Geometry check sheet. Reference: the model listing, model coordinates, mm. Face numbers are marked on the shaded views. A direction names the side the tool comes from. Round coordinates to 2 decimals unless told otherwise and drop trailing zeros. Loops run counter-clockwise (first coordinate to the right, second up) from the corner with the lowest first, then second, coordinate; pieces in that order, holes last. Notation, with made-up numbers: M 77,-33.5 L 133,-33.5 A24 cw 133,-21.5 Z; hole C -24,23 d5. An arc over 180 degrees is marked long. Use one line per item in the form item = value. Start each with the question number.
1. Cross-section at C-C (z = -2.5). Record the boundary of the cut face in (x, y).
2. Cross-section at B-B (y = 3.5). Record the boundary of the cut face in (x, z).
3. Set-up check for the marked faces 1 and 2: record each of +Z, -Z, +X, -X, +Y, -Y from which the full face is reachable in a straight line by a thin tool's end or side.
4. Go/stop test with flat-tipped pins: pin 1 (1.5 mm diameter, centred on x = 26, y = 11.5, fed in from -Z); pin 2 (6 mm diameter, centred on x = 131.5, z = -43.5, fed in from -Y); pin 3 (4 mm diameter, centred on x = 185.5, y = 12.7, fed in from +Z); pin 4 (2 mm diameter, centred on x = 58.5, y = -24, fed in from -Z). Record where each tip stops, or that it passes through.
5. Material ranges on line 1 (X direction, y = 12, z = 3); line 2 (X direction, y = -23, z = -42); line 3 (Y direction, x = 44.5, z = -7), recorded low to high.
6. Cross-section at A-A (x = 93). Record the boundary of the cut face in (y, z), then the cut area to 3 significant figures.
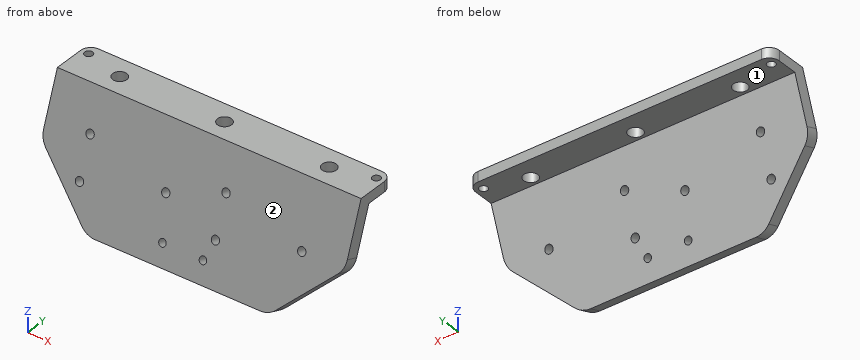
Autodesk Inventor part; units mm, degrees
ref_plane "YZ Plane" through (0, 0, 0) normal (1, 0, 0) x (0, 1, 0)
ref_plane "XZ Plane" through (0, 0, 0) normal (0, 1, 0) x (-1, 0, 0)
ref_plane "XY Plane" through (0, 0, 0) normal (0, 0, 1) x (1, 0, 0)
sketch "Sketch1" plane through (0, 0, 0) normal (0, 0, 1) x (1, 0, 0)
  line L0 (0, 0) -> (190.5, 0)
  line L1 (190.5, 0) -> (190.5, 19.05)
  line L2 (190.5, 19.05) -> (0, 19.05)
  line L3 (0, 19.05) -> (0, 0)
  dimension "d0" = 190.5
  dimension "d1" = 19.05
extrude "Extrusion1" add sketch "Sketch1" along normal blind 6.35
sketch "Sketch2" plane through (0, 0, 6.35) normal (0, 0, 1) x (1, 0, 0)
  circle A0 centre (5.0038, 12.7) radius 2.5527
  circle A1 centre (185.4962, 12.7) radius 2.5527
  line L0 (0, 19.05) -> (0, 0)
  line L1 (0, 0) -> (190.5, 0)
  point P0 (0, 9.525)
  point P1 (0, 9.525)
  dimension "d4" = 5.1054
  dimension "d5" = 5.1054
  dimension "d6" = 180.4924
  dimension "d10" = 5.0038
  dimension "d11" = 12.7
extrude "Extrusion2" cut sketch "Sketch2" against normal blind 6.35
fillet "Fillet1" radius 6.35 2 edges at (190.5, 19.05, 3.175) (0, 19.05, 3.175)
sketch "Sketch3" plane through (190.5, 0, 6.35) normal (1, 0, 0) x (0, 0, -1)
  line L0 (0, -6.35) -> (71.6046, -32.4119)
  line L1 (0, 0) -> (76.2, 0) construction
  line L2 (6.35, 12.7) -> (6.35, 0)
  line L3 (6.35, 0) -> (0, 0)
  line L4 (6.35, 0) -> (74.3882, -24.7639)
  line L5 (6.35, 0) -> (78.7548, 0) construction
  line L6 (74.3882, -24.7639) -> (71.6046, -32.4119)
  line L7 (0, 0) -> (0, 12.7)
  line L8 (0, 0) -> (0, -6.35)
  dimension "d13" = 76.2
  dimension "d14" = 20
  dimension "d17" = 20
  dimension "d18" = 6.35
extrude "Extrusion3" add sketch "Sketch3" against normal up to surface (190.5 mm away)
chamfer "Chamfer1" distance 38.1 angle 45 2 edges at (0, -28.5879, -66.6464) (190.5, -28.5879, -66.6464)
fillet "Fillet2" radius 12.7 4 edges at (38.1, -28.5879, -66.6464) (0, -15.5569, -30.8441) (152.4, -28.5879, -66.6464) (190.5, -15.5569, -30.8441)
sketch "Sketch5" plane through (0, 0, 6.35) normal (0, 0, 1) x (1, 0, 0)
  circle A0 centre (160.9621, 6.1265) radius 4.445
  circle A1 centre (185.4962, 12.7) radius 2.5527
  line L0 (185.4962, 12.7) -> (176.5159, 21.6803)
  line L1 (185.4962, 12.7) -> (198.1962, 12.7) construction
  line L2 (176.5159, 21.6803) -> (160.9621, 6.1265)
  line L3 (160.9621, 6.1265) -> (95.2523, 6.1265)
  line L4 (95.2523, 6.1265) -> (29.5425, 6.1265)
  circle A2 centre (29.5425, 6.1265) radius 4.445
  circle A3 centre (95.2523, 6.1265) radius 4.445
  point P0 (0, 0)
  dimension "d24" = 8.89
  dimension "d25" = 12.7
  dimension "d26" = 135
  dimension "d27" = 21.9964
  dimension "d30" = 65.7098
  dimension "d31" = 65.7098
  dimension "d32" = 8.89
  dimension "d33" = 8.89
extrude "Extrusion4" cut sketch "Sketch5" against normal blind 25.4 contours A0 L3 L2 | L2 L3 A0 | A3 L4 L3 | L3 L4 A3 | A2
sketch "Sketch6" plane through (0, -6.35, 6.35) normal (0, -0.9396926, 0.3420201) x (1, 0, 0)
  circle A0 centre (163.322, -38.354) radius 2.54
  line L0 (190.5, 0) -> (190.5, -32.8395)
  line L1 (147.1395, -76.2) -> (43.3605, -76.2)
  circle A1 centre (112.522, -51.054) radius 2.54
  circle A2 centre (112.522, -25.654) radius 2.54
  circle A3 centre (78.0288, -38.354) radius 2.54
  circle A4 centre (27.2288, -25.654) radius 2.54
  circle A5 centre (27.2288, -51.054) radius 2.54
  point P0 (0, -3.7952)
  dimension "d34" = 27.178
  dimension "d35" = 37.846
  dimension "d36" = 5.08
  dimension "d39" = 5.08
  dimension "d40" = 12.7
  dimension "d41" = 50.8
  dimension "d42" = 5.08
  dimension "d43" = 50.8
  dimension "d44" = 12.7
  dimension "d45" = 85.2932
  dimension "d46" = 5.08
  dimension "d47" = 5.08
  dimension "d48" = 5.08
  dimension "d51" = 50.8
  dimension "d52" = 50.8
extrude "Extrusion5" cut sketch "Sketch6" against normal blind 25.4
sketch "Sketch8" plane through (0, -6.35, 6.35) normal (0, -0.9396926, 0.3420201) x (1, 0, 0)
  line L0 (147.1395, -76.2) -> (43.3605, -76.2)
  line L1 (95.25, -76.2) -> (95.25, -63.5)
  line L2 (95.25, -63.5) -> (82.55, -63.5)
  line L3 (95.25, -63.5) -> (107.95, -63.5)
  point P0 (0, -3.7952)
  dimension "d58" = 12.7
  dimension "d59" = 12.7
  dimension "d60" = 12.7
hole "Hole1" at (82.55, -28.0683, -53.3205) at (107.95, -28.0683, -53.3205) direction (0, 0.9396926, -0.3420201) diameter 4.572 end through all
equation "\"d5\" = d4"
properties part number "Module_SPM_Mount_2.0_SMM"
Reported:
q1.outline = M 0,-9.57 L 190.5,-9.57 L 190.5,-0.91 L 0,-0.91 Z
q2.outline = M 0,0 L 25.96,0 L 25.96,6.35 L 0,6.35 Z; M 33.13,0 L 91.67,0 L 91.67,6.35 L 33.13,6.35 Z; M 98.84,0 L 157.38,0 L 157.38,6.35 L 98.84,6.35 Z; M 164.55,0 L 190.5,0 L 190.5,6.35 L 164.55,6.35 Z
q3.face_1 = -Z, +X, -X, +Y
q3.face_2 = +Z, +X, -X, -Y
q4.pin_1 = 0
q4.pin_2 = -25.59
q4.pin_3 = through
q4.pin_4 = -68.04
q5.line_1 = 0 to 2.55, 7.46 to 183.04, 187.95 to 190.5
q5.line_2 = 13.03 to 24.69, 29.77 to 109.98, 115.06 to 177.47
q5.line_3 = -11.21 to -2.55
q6.outline = M -32.41,-65.25 L -24.76,-68.04 L 0,0 L 2.29,0 L 2.29,6.35 L -6.35,6.35 Z; M 9.96,0 L 19.05,0 L 19.05,6.35 L 9.96,6.35 Z
q6.area = 697 mm²
